```python
from build123d import *

# Parameters (mm, degrees)
SKETCH3_R          = 2.032
CUT_EXTRUDE1_DEPTH = 5.318


with BuildPart() as part:
    # Sketch2 → Revolve1 (revolve)
    with BuildSketch(Plane.XY):
        Polygon((3.175, 0), (4.318, 0), (4.318, 18.288), (2.159, 18.288), (2.159, 17.018), (2.921, 17.018), (2.921, 12.7), (3.175, 12.7), align=None)
    revolve(axis=Axis((0, 0, 0), (0, 1, 0)))

    # Sketch3 → Cut-Extrude1 (cut, through all)
    with BuildSketch(Plane.XY):
        with Locations((0, 8.128)):
            Circle(SKETCH3_R)
    extrude(amount=-CUT_EXTRUDE1_DEPTH, mode=Mode.SUBTRACT)


solid = part.part
```
Geometry check sheet. Reference: the model listing, model coordinates, mm. A direction names the side the tool comes from. Give positions to 0.01 mm unless a question says otherwise; leave off trailing zeros. Order: outer loops, then holes, each group sorted by start corner. A loop starts at its lowest first (then second) coordinate and runs counter-clockwise, first axis right, second up.
1. Section check D-D, the plane y = 3.75. Enter the section's corners in (x, z) (3 decimals), and give its area (3 significant figures).
2. Access from +Z, -Z, +X, -X, +Y, -Y to the whole of each face (thin tool, end or side, straight path). Record for faces 1 (the face through (3, 0, -2)), 2 (the face through (-0.44, 6.144, -3.366)), 3 (the face through (-0.633, 14.829, 2.852)).
3. Section check B-B, the plane x = 0. Enter the section's corners in (y, z) (3 decimals).
4. Gauge pin test, flat ends, axial feed: pin 1 Ø3 at (x, z) = (1.5, 0.5) entering from -Y; pin 2 Ø3.5 at (x, y) = (0, 8.128) entering from -Z; pin 3 Ø3.5 at (x, z) = (0, 0) entering from +Y; pin 4 Ø1.9 at (x, z) = (-1, 1.5) entering from -Y. Record the tip position at first contact, or that the pin passes through.
5. Release check for a two-part mould opening along X. For faces 4 (the face through (-0.936, 9.272, 4.215)), 5 (the face through (2, 18.288, 2)), 6 (the face through (-0.69, 6.26, 3.1)) record: pulls with the +X half, pulls with the -X half, needs draft (parallel to the pull), parting line crosses it, or undercut.
6. Section check C-C, the plane x = -2.5. Enter the section's corners in (y, z).
7. Section check A-A, the plane z = 0. Enter the section's corners in (x, y) (3 decimals), and give its area (3 significant figures).
8. Thickness scan on L1, parallel to Z at x = 0, y = 17.9; L2, parallel to Z at x = 0, y = 3.75 (3 decimals); L3, parallel to X at y = 16.1, z = 0. Record the ranges inside material, lowest first.
Values follow:
1. outline: circle Ø8.636 at (0, 0); hole circle Ø6.35 at (0, 0)
1. area: 26.9 mm2
2. face 1: +Z, -Z, +X, -X, -Y
2. face 2: -Z
2. face 3: -Y
3. outline: (0, -4.318) - (6.096, -4.318) - (6.096, -3.175) - (0, -3.175) - close; (0, 3.175) - (12.7, 3.175) - (12.7, 2.921) - (17.018, 2.921) - (17.018, 2.159) - (18.288, 2.159) - (18.288, 4.318) - (0, 4.318) - close; (10.16, -4.318) - (18.288, -4.318) - (18.288, -2.159) - (17.018, -2.159) - (17.018, -2.921) - (12.7, -2.921) - (12.7, -3.175) - (10.16, -3.175) - close
4. pin 1: stops at y = 12.7
4. pin 2: stops at z = 2.65
4. pin 3: passes through
4. pin 4: stops at y = 17.02
5. face 4: parting line crosses it
5. face 5: needs draft
5. face 6: undercut
6. outline: (0, -3.52) - (18.29, -3.52) - (18.29, 3.52) - (0, 3.52) - (0, 1.96) - (12.7, 1.96) - (12.7, 1.51) - (17.02, 1.51) - (17.02, -1.51) - (12.7, -1.51) - (12.7, -1.96) - (0, -1.96) - close
7. outline: (-4.318, 0) - (-3.175, 0) - (-3.175, 12.7) - (-2.921, 12.7) - (-2.921, 17.018) - (-2.159, 17.018) - (-2.159, 18.288) - (-4.318, 18.288) - close; (2.159, 17.018) - (2.921, 17.018) - (2.921, 12.7) - (3.175, 12.7) - (3.175, 0) - (4.318, 0) - (4.318, 18.288) - (2.159, 18.288) - close
7. area: 46.6 mm2
8. L1: z = -4.32 to -2.16, 2.16 to 4.32
8. L2: z = -4.318 to -3.175, 3.175 to 4.318
8. L3: x = -4.32 to -2.92, 2.92 to 4.32
